```python
from build123d import *

# Parameters (mm, degrees)
F1_DEPTH = 30


with BuildPart() as f1:
    # F0 (on Top) → F1 (new body)
    with BuildSketch(Plane.XY):
        with BuildLine():
            ThreePointArc((3.752684, -4.721397), (5.320047, -7.70051), (8.180264, -5.925433))
            Line((8.180264, -5.925433), (10.322446, 4.071413))
            ThreePointArc((10.322446, 4.071413), (9.722037, 6.586033), (7.389038, 7.7))
            Line((7.389038, 7.7), (-7.389038, 7.7))
            ThreePointArc((-7.389038, 7.7), (-9.722037, 6.586033), (-10.322446, 4.071413))
            Line((-10.322446, 4.071413), (-8.180264, -5.925433))
            Line((-8.180264, -5.925433), (-8.164181, -6.000488))
            ThreePointArc((-8.164181, -6.000488), (-7.982367, -6.506508), (-7.688034, -6.956488))
            ThreePointArc((-7.688034, -6.956488), (-4.787716, -7.481058), (-3.752684, -4.721397))
            ThreePointArc((-3.752684, -4.721397), (-4.017831, -4.328982), (-4.242095, -3.911851))
            ThreePointArc((-4.242095, -3.911851), (-4.247654, -3.905916), (-4.253234, -3.9))
            ThreePointArc((-4.253234, -3.9), (0, 2.8), (4.253234, -3.9))
            ThreePointArc((4.253234, -3.9), (4.247654, -3.905916), (4.242095, -3.911851))
            ThreePointArc((4.242095, -3.911851), (4.017831, -4.328982), (3.752684, -4.721397))
        make_face()
        with BuildLine():
            Line((-8.164181, -6.000488), (-8.180264, -5.925433))
            ThreePointArc((-8.180264, -5.925433), (-8.172536, -5.963027), (-8.164181, -6.000488))
        make_face()
        with BuildLine():
            ThreePointArc((-7.688034, -6.956488), (-7.982367, -6.506508), (-8.164181, -6.000488))
            ThreePointArc((-8.164181, -6.000488), (-7.986414, -6.508524), (-7.688034, -6.956488))
        make_face()
    extrude(amount=F1_DEPTH)


solid = f1.part
```
Input: part model. Units: mm. Frame: model coordinates. A direction names the side the tool comes from. Give positions to 0.01 mm unless a question says otherwise; leave off trailing zeros. Order: outer loops, then holes, each group sorted by start corner. A loop starts at its lowest first (then second) coordinate and runs counter-clockwise, first axis right, second up. Notation, with made-up numbers: (3, 52) - (30, 52) arc R21 cw to (30, 58) - close; hole circle Ø7 at (63, 76). An arc over 180 degrees is marked (long way). Put each result on its own line as item: value.
Item 1: Contact query for flat-ended pins moving along their axis: pin 1 (8 mm diameter, centred on y = -5.5, z = 18.5, fed in from +X); pin 2 (4 mm diameter, centred on y = -5, z = 16.5, fed in from -X). Output: stop coordinate, or through.
Found:
pin 1: stops at x = 9.13
pin 2: stops at x = -8.81
Item 2: Section query A-A, the plane y = -1.9. Return loops of the section in (x, z), then the cut area to 3 significant figures.
Found:
outline: (-9.04, 0) - (-4.7, 0) - (-4.7, 30) - (-9.04, 30) - close; (4.7, 0) - (9.04, 0) - (9.04, 30) - (4.7, 30) - close
area: 261 mm^2
Item 3: Access query for faces 1 (the cylindrical face through (-4.014, -4.335, 14.79)), 2 (the flat face through (0, 7.7, 15)). Directions: +Z, -Z, +X, -X, +Y, -Y. A direction counts if a zero-diameter tool reaches every point of the face in a straight line with its end or side. Return the directions, or none.
Found:
face 1: +Z, -Z
face 2: +Z, -Z, +X, -X, +Y
Item 4: Draft query along Y for faces 3 (the flat face through (0, 4, 0)), 4 (the flat face through (9.236, -0.997, 14.79)), 5 (the cylindrical face through (4.021, -4.323, 14.79)), 6 (the cylindrical face through (-0.1, 2.8, 14.8)). Return one class per face: +Y half, -Y half, draft (parallel to the pull), parting line (faces both ways), or undercut.
Found:
face 3: draft
face 4: -Y half
face 5: undercut
face 6: undercut
Item 5: Section query D-D, the plane y = -6.5. Return loops of the section in (x, z), then the cut area to 3 significant figures.
Found:
outline: (-7.99, 0) - (-3.86, 0) - (-3.86, 30) - (-7.99, 30) - close; (3.86, 0) - (7.99, 0) - (7.99, 30) - (3.86, 30) - close
area: 248 mm^2
Item 6: Section query C-C, the plane x = 0. Return loops of the section in (y, z).
Found:
outline: (2.8, 0) - (7.7, 0) - (7.7, 30) - (2.8, 30) - close
Item 7: Ray query, L1, parallel to X at y = -3.75, z = 6.25; L2, parallel to X at y = -1.9, z = 8.5; L3, parallel to Y at x = 0, z = 10.75. Return the intervals inside material, ascending. Write a range as from..to.
Found:
L1: x = -8.65..-4.32, 4.32..8.65
L2: x = -9.04..-4.7, 4.7..9.04
L3: y = 2.8..7.7
